from build123d import *

# Parameters (mm, degrees)
BOSS_EXTRUDE1_DEPTH = 8
SKETCH3_R           = 4
BOSS_EXTRUDE2_DEPTH = 14


with BuildPart() as part:
    # Sketch2 → Boss-Extrude1 (new body)
    with BuildSketch(Plane(origin=(0, 0, 0), x_dir=(1, 0, 0), z_dir=(0, 1, 0))):
        with BuildLine():
            Line((-5, 6.244997998), (-5, 39.101020514))
            ThreePointArc((-5, 39.101020514), (-6.480740698, 41.354248689), (-7, 44))
            Line((-7, 44), (-7, 67))
            ThreePointArc((-7, 67), (-6.84274311, 68.475420866), (-6.378038076, 69.884550276))
            Line((-6.378038076, 69.884550276), (0, 98))
            Line((0, 98), (6.378038076, 69.884550276))
            ThreePointArc((6.378038076, 69.884550276), (6.84274311, 68.475420866), (7, 67))
            Line((7, 67), (7, 44))
            ThreePointArc((7, 44), (6.480740698, 41.354248689), (5, 39.101020514))
            Line((5, 39.101020514), (5, 6.244997998))
            ThreePointArc((5, 6.244997998), (0, -8), (-5, 6.244997998))
        make_face()
        with BuildLine():
            Line((-3, 67), (-3, 44))
            ThreePointArc((-3, 44), (0, 41), (3, 44))
            Line((3, 44), (3, 67))
            ThreePointArc((3, 67), (0, 70), (-3, 67))
        make_face(mode=Mode.SUBTRACT)
    extrude(amount=BOSS_EXTRUDE1_DEPTH)

    # Sketch3 → Boss-Extrude2 (add)
    with BuildSketch(Plane.XZ):
        Circle(SKETCH3_R)
    extrude(amount=BOSS_EXTRUDE2_DEPTH)


solid = part.part
Work out the finished part from the listing and answer in its coordinate system (mm). A direction names the side the tool comes from. Round coordinates to 2 decimals unless told otherwise and drop trailing zeros. Loops run counter-clockwise (first coordinate to the right, second up) from the corner with the lowest first, then second, coordinate; pieces in that order, holes last. Notation, with made-up numbers: (57, 30.25) - (114, 30.25) arc R24 cw to (114, 53.25) - close; hole circle Ø7 at (79, 80.25). An arc over 180 degrees is marked (long way). Use one line per item in the form item = value. Start each with the question number.
(1) Consider line 1 (Y direction, x = 4, z = -24); line 2 (X direction, y = 0.5, z = -68); line 3 (X direction, y = 3.25, z = -69). Determine where each line is inside the solid, lowest interval first.
(2) Find section B-B on y = 2.25. Determine the outline of the cut face in (x, z) (3 decimals), and give its area (3 significant figures).
(3) Find section A-A on z = -57. Determine the outline of the cut face in (x, y), and give its area (3 significant figures).
(4) Which of the six approach directions +Z, -Z, +X, -X, +Y, -Y give full straight-line access (tool end or side, diameter ignored) to faces 1 (the face through (-6.466, 3.944, -41.319)), 2 (the face through (3, 4, -55)), 3 (the face through (7, 4, -56)), 4 (the face through (-7, 4, -55)), 5 (the face through (5, 4, -23))?
(5) Find section C-C on z = 0. Determine the outline of the cut face in (x, y), and give its area (3 significant figures).
(6) Find section D-D on y = -1.75. Determine the outline of the cut face in (x, z), and give its area (3 significant figures).
(7) Flat-ended cylindrical pins translate along their axes: P1, Ø4, axis at y = 5, z = -51, coming from the +X side; P2, Ø2.5, axis at y = 5.5, z = -26.5, coming from the +X side; P3, Ø4, axis at x = 2, y = -10.5, coming from the +Z side. Find the tip coordinate at first contact, or state that the pin passes through.
(8) Determine the mould class of faces 6 (the face through (0, 4, -41)), 7 (the face through (-3.234, 3.944, -83.745)), 8 (the face through (3.144, 3.944, -84.139)) for opening direction X: +X half, -X half, draft (parallel to the pull), parting line (faces both ways), or undercut.
Answer list:
q1.line_1 = 0 to 8
q1.line_2 = -6.93 to -2.83, 2.83 to 6.93
q1.line_3 = -6.71 to -2.24, 2.24 to 6.71
q2.outline = (-7, -67) arc R7 ccw to (-6.378, -69.885) - (0, -98) - (6.378, -69.885) arc R7 ccw to (7, -67) - (7, -44) arc R7 ccw to (5, -39.101) - (5, -6.245) arc R8 ccw (long way) to (-5, -6.245) - (-5, -39.101) arc R7 ccw to (-7, -44) - close; hole (-3, -67) arc R3 ccw to (3, -67) - (3, -44) arc R3 ccw to (-3, -44) - close
q2.area = 954 mm^2
q3.outline = (-7, 0) - (-3, 0) - (-3, 8) - (-7, 8) - close; (3, 0) - (7, 0) - (7, 8) - (3, 8) - close
q3.area = 64.0 mm^2
q4.face_1 = -X, +Y, -Y
q4.face_2 = +Y, -Y
q4.face_3 = -Z, +X, +Y, -Y
q4.face_4 = -Z, -X, +Y, -Y
q4.face_5 = +X, +Y, -Y
q5.outline = (-8, 0) - (-4, 0) - (-4, -14) - (4, -14) - (4, 0) - (8, 0) - (8, 8) - (-8, 8) - close
q5.area = 240 mm^2
q6.outline = circle Ø8 at (0, 0)
q6.area = 50.3 mm^2
q7.P1 = 7
q7.P2 = 5
q7.P3 = 4
q8.face_6 = undercut
q8.face_7 = -X half
q8.face_8 = +X half
